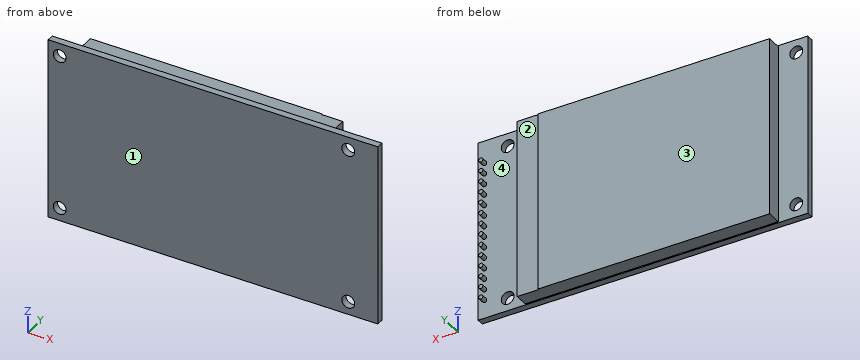
```python
from build123d import *

# Parameters (mm, degrees)
CROQUIS1_W              = 77.1
CROQUIS1_H              = 42.7
SALIENTE_EXTRUIR1_DEPTH = 1.6
CROQUIS2_W              = 59.2
CROQUIS2_H              = 42.2
SALIENTE_EXTRUIR2_DEPTH = 3.4
CORTAR_EXTRUIR2_REACH   = 46.35
CROQUIS4_R              = 1.5
CUT_EXTRUDE1_DEPTH      = 45.350028185
CUT_EXTRUDE1_DEPTH_BACK = 0.25
CROQUIS3_R              = 0.5
BOSS_EXTRUDE1_DEPTH     = 1.5


with BuildPart() as part:
    # Croquis1 → Saliente-Extruir1 (new body)
    with BuildSketch(Plane(origin=(0, 0, 0), x_dir=(1, 0, 0), z_dir=(0, 1, 0))):
        Rectangle(CROQUIS1_W, CROQUIS1_H)
    extrude(amount=SALIENTE_EXTRUIR1_DEPTH)

    # Croquis2 → Saliente-Extruir2 (add)
    with BuildSketch(Plane(origin=(0, 1.6, 0), x_dir=(1, 0, 0), z_dir=(0, 1, 0))):
        with Locations((-2.05, 0)):
            Rectangle(CROQUIS2_W, CROQUIS2_H)
    extrude(amount=SALIENTE_EXTRUIR2_DEPTH)

    # Croquis4 → Cortar-Extruir2 (cut, up to next)
    with BuildSketch(Plane.XZ, mode=Mode.PRIVATE) as cortar_extruir2_sk1:
        with Locations(Location((-35.85, 18.3, 0), (0, 0, 270))):
            Circle(CROQUIS4_R)
    cortar_extruir2_tool1 = extrude(cortar_extruir2_sk1.sketch, amount=-CORTAR_EXTRUIR2_REACH, mode=Mode.PRIVATE) & part.part
    # Croquis4 → Cortar-Extruir2 (cut, up to next)
    with BuildSketch(Plane.XZ, mode=Mode.PRIVATE) as cortar_extruir2_sk2:
        with Locations(Location((31.65, 18.3, 0), (0, 0, 270))):
            Circle(CROQUIS4_R)
    cortar_extruir2_tool2 = extrude(cortar_extruir2_sk2.sketch, amount=-CORTAR_EXTRUIR2_REACH, mode=Mode.PRIVATE) & part.part
    # Croquis4 → Cortar-Extruir2 (cut, up to next)
    with BuildSketch(Plane.XZ, mode=Mode.PRIVATE) as cortar_extruir2_sk3:
        with Locations(Location((31.65, -18.3, 0), (0, 0, 270))):
            Circle(CROQUIS4_R)
    cortar_extruir2_tool3 = extrude(cortar_extruir2_sk3.sketch, amount=-CORTAR_EXTRUIR2_REACH, mode=Mode.PRIVATE) & part.part
    # Croquis4 → Cortar-Extruir2 (cut, up to next)
    with BuildSketch(Plane.XZ, mode=Mode.PRIVATE) as cortar_extruir2_sk4:
        with Locations(Location((-35.85, -18.3, 0), (0, 0, 270))):
            Circle(CROQUIS4_R)
    cortar_extruir2_tool4 = extrude(cortar_extruir2_sk4.sketch, amount=-CORTAR_EXTRUIR2_REACH, mode=Mode.PRIVATE) & part.part
    add(cortar_extruir2_tool1.solids().sort_by_distance((-35.85, 0, 18.3))[0], mode=Mode.SUBTRACT)
    add(cortar_extruir2_tool2.solids().sort_by_distance((31.65, 0, 18.3))[0], mode=Mode.SUBTRACT)
    add(cortar_extruir2_tool3.solids().sort_by_distance((31.65, 0, -18.3))[0], mode=Mode.SUBTRACT)
    add(cortar_extruir2_tool4.solids().sort_by_distance((-35.85, 0, -18.3))[0], mode=Mode.SUBTRACT)

    # Sketch3 → Cut-Extrude1 (cut, two sides: drawn at the far end of the back side and taken through both)
    with BuildSketch(Plane(origin=(0, 5, 0), x_dir=(1, 0, 0), z_dir=(0, 1, 0)).offset(-CUT_EXTRUDE1_DEPTH_BACK)):
        Polygon((22.55, 179.899832697), (22.55, 21.10051324), (22.55, -21.101140947), (22.55, -179.900460404), (340.148638914, -179.900460404), (340.148638914, 179.899832697), align=None)
    extrude(amount=CUT_EXTRUDE1_DEPTH + CUT_EXTRUDE1_DEPTH_BACK, mode=Mode.SUBTRACT)

    # Croquis3 → Boss-Extrude1 (add)
    with BuildSketch(Plane(origin=(0, 1.6, 0), x_dir=(1, 0, 0), z_dir=(0, 1, 0))):
        with Locations(Location((37.05, -15.923235508, 0), (0, 0, 270))):
            Circle(CROQUIS3_R)
        with Locations(Location((37.05, -13.383235508, 0), (0, 0, 270))):
            Circle(CROQUIS3_R)
        with Locations(Location((37.05, -10.843235508, 0), (0, 0, 270))):
            Circle(CROQUIS3_R)
        with Locations(Location((37.05, -8.303235508, 0), (0, 0, 270))):
            Circle(CROQUIS3_R)
        with Locations(Location((37.05, -5.763235508, 0), (0, 0, 270))):
            Circle(CROQUIS3_R)
        with Locations(Location((37.05, -3.223235508, 0), (0, 0, 270))):
            Circle(CROQUIS3_R)
        with Locations(Location((37.05, -0.683235508, 0), (0, 0, 270))):
            Circle(CROQUIS3_R)
        with Locations(Location((37.05, 1.856764492, 0), (0, 0, 270))):
            Circle(CROQUIS3_R)
        with Locations(Location((37.05, 4.396764492, 0), (0, 0, 270))):
            Circle(CROQUIS3_R)
        with Locations(Location((37.05, 6.936764492, 0), (0, 0, 270))):
            Circle(CROQUIS3_R)
        with Locations(Location((37.05, 9.476764492, 0), (0, 0, 270))):
            Circle(CROQUIS3_R)
        with Locations(Location((37.05, 12.016764492, 0), (0, 0, 270))):
            Circle(CROQUIS3_R)
        with Locations(Location((37.05, 14.556764492, 0), (0, 0, 270))):
            Circle(CROQUIS3_R)
        with Locations(Location((37.05, 17.096764492, 0), (0, 0, 270))):
            Circle(CROQUIS3_R)
    extrude(amount=BOSS_EXTRUDE1_DEPTH)


solid = part.part
```
Could you check a few things on this model? Use its own coordinates, in mm. Face numbers are marked on the shaded views. A direction names the side the tool comes from. Round coordinates to 2 decimals unless told otherwise and drop trailing zeros. Loops run counter-clockwise (first coordinate to the right, second up) from the corner with the lowest first, then second, coordinate; pieces in that order, holes last. Notation, with made-up numbers: (40.25, -22) -> (92.25, -22) arc R24 cw to (92.25, -9) -> close; hole circle Ø7 at (30.25, -30). An arc over 180 degrees is marked (long way). One line per question, with ' | ' between items.
(1) If we section it at B-B on z = 18.3: List the corners of the cut face in (x, y) for me.
Model answer:
outline: (-38.55, 0) -> (-37.35, 0) -> (-37.35, 1.6) -> (-38.55, 1.6) -> close; (-34.35, 0) -> (30.15, 0) -> (30.15, 1.6) -> (27.55, 1.6) -> (27.55, 4.75) -> (22.55, 4.75) -> (22.55, 5) -> (-31.65, 5) -> (-31.65, 1.6) -> (-34.35, 1.6) -> close; (33.15, 0) -> (38.55, 0) -> (38.55, 1.6) -> (33.15, 1.6) -> close
(2) If we section it at C-C on x = 23.5: List the corners of the cut face in (y, z) for me, and give its area (3 significant figures).
Model answer:
outline: (0, -21.35) -> (1.6, -21.35) -> (1.6, -21.1) -> (4.75, -21.1) -> (4.75, 21.1) -> (1.6, 21.1) -> (1.6, 21.35) -> (0, 21.35) -> close | area: 201 mm^2
(3) For pin 1 Ø0.8 at (x, z) = (37, 0.5) entering from +Y; pin 2 Ø2.5 at (y, z) = (4, -8.5) entering from -X; pin 3 Ø1.5 at (y, z) = (3.5, -3.5) entering from +X, each with a flat end and sliding along its axis, tell me the tip position at first contact or that it passes through.
Model answer:
pin 1: stops at y = 3.1 | pin 2: stops at x = -31.65 | pin 3: stops at x = 37.48
(4) Thinking about a two-plate mould opening in X: for the marked faces 3 and 4, which applies, released by +X, released by -X, zero draft, split by the parting line, or undercut?
Model answer:
face 3: zero draft | face 4: undercut
(5) If I drill on probe 1 along X at (y, z) = (0.8, -18.3); probe 2 along Z at (x, y) = (4, 3.8); probe 3 along X at (y, z) = (1.15, -17.5), over which ranges is the centre line in solid material (lowest first)?
Model answer:
probe 1: x = -38.55 to -37.35, -34.35 to 30.15, 33.15 to 38.55 | probe 2: z = -21.1 to 21.1 | probe 3: x = -38.55 to -37.12, -34.58 to 30.38, 32.92 to 38.55
(6) If we section it at A-A on x = 31.65: List the corners of the cut face in (y, z) for me, and give its area (3 significant figures).
Model answer:
outline: (0, -21.35) -> (1.6, -21.35) -> (1.6, -19.8) -> (0, -19.8) -> close; (0, -16.8) -> (1.6, -16.8) -> (1.6, 16.8) -> (0, 16.8) -> close; (0, 19.8) -> (1.6, 19.8) -> (1.6, 21.35) -> (0, 21.35) -> close | area: 58.7 mm^2
(7) For the marked faces 1 and 2, which set-ups out of +Z, -Z, +X, -X, +Y, -Y let a thin tool reach every point of the face, with its end or its side?
Model answer:
face 1: +Z, -Z, +X, -X, -Y | face 2: +Z, -Z, +X, +Y
